```python
from build123d import *

# Parameters (mm, degrees)
SKETCH1_W                                   = 190.5
SKETCH1_H                                   = 190.5
SKETCH1_R                                   = 9.525
BOSS_EXTRUDE1_DEPTH                         = 25.4
SKETCH1_3_R                                 = 9.525
BOSS_EXTRUDE2_DEPTH                         = 25.4
SKETCH3_W                                   = 139.7
SKETCH3_H                                   = 139.7
BOSS_EXTRUDE3_DEPTH                         = 203.2
FILLET1_RADIUS                              = 69.85
FILLET1_LENGTH                              = 139.7
CBORE_FOR_1_1_2_HEAVY_HEX_BOLT1_D           = 38.89248
CBORE_FOR_1_1_2_HEAVY_HEX_BOLT1_CBORE_D     = 88.9
CBORE_FOR_1_1_2_HEAVY_HEX_BOLT1_CBORE_DEPTH = 26.3144
FILLET2_R                                   = 12.7


with BuildPart() as part:
    # Sketch1 → Boss-Extrude1 (new body)
    # profile 1 of 5: a face of its own
    with BuildSketch(Plane(origin=(0, 0, 0), x_dir=(1, 0, 0), z_dir=(0, 1, 0))):
        Rectangle(SKETCH1_W, SKETCH1_H)
        with Locations((-57.15, -57.15)):
            Circle(SKETCH1_R, mode=Mode.SUBTRACT)
        with Locations((57.15, -57.15)):
            Circle(SKETCH1_R, mode=Mode.SUBTRACT)
        with Locations((57.15, 57.15)):
            Circle(SKETCH1_R, mode=Mode.SUBTRACT)
        with Locations((-57.15, 57.15)):
            Circle(SKETCH1_R, mode=Mode.SUBTRACT)
    # profile 2 of 5: a face of its own
    with BuildSketch(Plane(origin=(0, 0, 0), x_dir=(1, 0, 0), z_dir=(0, 1, 0))):
        with Locations((-57.15, -57.15)):
            Circle(SKETCH1_R)
    # profile 3 of 5: a face of its own
    with BuildSketch(Plane(origin=(0, 0, 0), x_dir=(1, 0, 0), z_dir=(0, 1, 0))):
        with Locations((-57.15, 57.15)):
            Circle(SKETCH1_R)
    # profile 4 of 5: a face of its own
    with BuildSketch(Plane(origin=(0, 0, 0), x_dir=(1, 0, 0), z_dir=(0, 1, 0))):
        with Locations((57.15, 57.15)):
            Circle(SKETCH1_R)
    # profile 5 of 5: a face of its own
    with BuildSketch(Plane(origin=(0, 0, 0), x_dir=(1, 0, 0), z_dir=(0, 1, 0))):
        with Locations((57.15, -57.15)):
            Circle(SKETCH1_R)
    extrude(amount=BOSS_EXTRUDE1_DEPTH)

    # Sketch1<3> → Boss-Extrude2 (add)
    with BuildSketch(Plane(origin=(0, 0, 0), x_dir=(1, 0, 0), z_dir=(0, 1, 0))):
        with Locations(Location((-57.15, 57.15, 0), (0, 0, 270))):
            Circle(SKETCH1_3_R)
        with Locations(Location((57.15, 57.15, 0), (0, 0, 270))):
            Circle(SKETCH1_3_R)
        with Locations(Location((57.15, -57.15, 0), (0, 0, 270))):
            Circle(SKETCH1_3_R)
        with Locations(Location((-57.15, -57.15, 0), (0, 0, 270))):
            Circle(SKETCH1_3_R)
    extrude(amount=-BOSS_EXTRUDE2_DEPTH)

    # Sketch3 → Boss-Extrude3 (add)
    with BuildSketch(Plane(origin=(0, 25.4, 0), x_dir=(1, 0, 0), z_dir=(0, 1, 0))):
        Rectangle(SKETCH3_W, SKETCH3_H)
    extrude(amount=BOSS_EXTRUDE3_DEPTH)

    # Fillet1: full round fillet: the end face becomes a half cylinder, R = half its width
    fillet1_face = Plane((0, 228.6, 0), x_dir=(-1, 0, 0), z_dir=(0, 1, 0))  # on the end face: x along it, z out of the body
    fillet1_slab = fillet1_face.offset(-FILLET1_RADIUS / 2) * Box(FILLET1_LENGTH, 2 * FILLET1_RADIUS, FILLET1_RADIUS, mode=Mode.PRIVATE)  # the body's end, R deep
    fillet1_round = Plane((0, 158.75, 0), x_dir=(0, 1, 0), z_dir=(-1, 0, 0)) * Cylinder(FILLET1_RADIUS, FILLET1_LENGTH, mode=Mode.PRIVATE)  # its axis R under the face
    add(fillet1_slab - fillet1_round, mode=Mode.SUBTRACT)

    # CBORE for 1-1/2 Heavy Hex Bolt1 (through all)
    with Locations(Plane(origin=(69.85, 0, 0), x_dir=(0, 0, 1), z_dir=(1, 0, 0))):
        with Locations((0, -158.75)):
            CounterBoreHole(CBORE_FOR_1_1_2_HEAVY_HEX_BOLT1_D / 2, CBORE_FOR_1_1_2_HEAVY_HEX_BOLT1_CBORE_D / 2, CBORE_FOR_1_1_2_HEAVY_HEX_BOLT1_CBORE_DEPTH)

    # Fillet2
    fillet2_edges = [part.edges().sort_by_distance(p)[0] for p in [
        (0, 25.4, -69.85),
        (-69.85, 25.4, 0),
        (0, 25.4, 69.85),
        (69.85, 25.4, 0),
        (69.85, 92.075, 69.85),
        (-69.85, 92.075, 69.85),
        (-69.85, 92.075, -69.85),
        (69.85, 92.075, -69.85),
        (69.85, 228.6, 0),
        (-69.85, 228.6, 0),
    ]]
    fillet(fillet2_edges, radius=FILLET2_R)


solid = part.part
```
Here's how the part is built. I have some questions about the finished solid (model axes, mm). A direction names the side the tool comes from. Coordinates: 2 decimals unless noted, no trailing zeros. Order: outer loops, then holes, each group sorted by start corner. A loop starts at its lowest first (then second) coordinate and runs counter-clockwise, first axis right, second up. Notation, with made-up numbers: (-38, 88.5) - (-33, 88.5) arc R18 ccw to (-33, 108.5) - close; hole circle Ø8 at (-28, 84). An arc over 180 degrees is marked (long way). One line per question, with ' | ' between items.
(1) Will these pins go through, and if not, where does the flat tip stop? pin 1 (12 mm diameter, centred on x = 14.5, y = 32.5, fed in from -Z); pin 2 (1.5 mm diameter, centred on x = -45, y = 101.5, fed in from +Z); pin 3 (2 mm diameter, centred on x = -37, z = -20.5, fed in from -Y).
Report:
pin 1: stops at z = -77.38 | pin 2: stops at z = 69.85 | pin 3: stops at y = 0
(2) Suppose I cut it at C-C on y = -7. List the corners of the cut face in (x, z) for me (3 decimals), and give its area (3 significant figures).
Report:
outline: circle Ø19.05 at (-57.15, -57.15); circle Ø19.05 at (-57.15, 57.15); circle Ø19.05 at (57.15, -57.15); circle Ø19.05 at (57.15, 57.15) | area: 1,140 mm2
(3) Suppose I cut it at B-B on y = 92.5. List the corners of the cut face in (x, z) for me.
Report:
outline: (-69.85, -57.15) arc R12.7 ccw to (-57.15, -69.85) - (57.15, -69.85) arc R12.7 ccw to (69.85, -57.15) - (69.85, 57.15) arc R12.7 ccw to (57.15, 69.85) - (-57.15, 69.85) arc R12.7 ccw to (-69.85, 57.15) - close
(4) If I drill on L1, parallel to Y at x = 13, z = 0; L2, parallel to X at y = 193, z = 33; L3, parallel to X at y = 159, z = -39, over which ranges is the centre line in solid material (lowest first)?
Report:
L1: y = 0 to 139.3, 178.2 to 228.6 | L2: x = -69.85 to 69.85 | L3: x = -69.85 to 43.54
(5) Suppose I cut it at A-A on x = -13. List the corners of the cut face in (y, z) for me.
Report:
outline: (0, -95.25) - (25.4, -95.25) - (25.4, -82.55) arc R12.7 cw to (38.1, -69.85) - (158.75, -69.85) arc R69.85 ccw to (158.75, 69.85) - (38.1, 69.85) arc R12.7 cw to (25.4, 82.55) - (25.4, 95.25) - (0, 95.25) - close; hole circle Ø38.89 at (158.75, 0)
(6) For faces 4 (the cylindrical face through (51.354, -12.522, 49.591)), 5 (the flat face through (-1, 98, 69.85)), 6 (the flat face through (69.85, 106, 1)), 7 (the cylindrical face through (-66.03, 97.58, -66.23)), which set-ups out of +Z, -Z, +X, -X, +Y, -Y let a thin tool reach every point of the face, with its end or its side?
Report:
face 4: -Y | face 5: +Z, +X, -X, +Y | face 6: +Z, -Z, +X, +Y | face 7: -Z, -X, +Y
(7) If we mould it in two halves opening along Y, with no side actions, what happens to faces 1 (the cylindrical face through (-73.67, 29.02, -0.8)), 2 (the cylindrical face through (-50.71, -12.52, 50.13)), 3 (the flat face through (43.536, 178, 9))? For each: pulls with the +Y half, pulls with the -Y half, needs draft (parallel to the pull), parting line crosses it, or undercut.
Report:
face 1: pulls with the +Y half | face 2: needs draft | face 3: undercut
(8) Suppose I cut it at D-D on x = 53. List the corners of the cut face in (y, z) for me.
Report:
outline: (-25.4, -65.72) - (0, -65.72) - (0, -95.25) - (25.4, -95.25) - (25.4, -82.55) arc R12.7 cw to (38.1, -69.85) - (158.75, -69.85) arc R69.85 ccw to (158.75, 69.85) - (38.1, 69.85) arc R12.7 cw to (25.4, 82.55) - (25.4, 95.25) - (0, 95.25) - (0, 65.72) - (-25.4, 65.72) - (-25.4, 48.58) - (0, 48.58) - (0, -48.58) - (-25.4, -48.58) - close; hole circle Ø88.9 at (158.75, 0)
